```python
from build123d import *

# Parameters (mm, degrees)
F0_W     = 101.6
F0_H     = 25.4
F1_DEPTH = 25.4
F2_DEPTH = 12.7
F3_DEPTH = 63.5
F4_R     = 5.08
F5_SIZE  = 5.08


with BuildPart() as f1:
    # F0 (on Front) → F1 (new body, symmetric)
    with BuildSketch(Plane.XZ):
        Rectangle(F0_W, F0_H)
    extrude(amount=F1_DEPTH, both=True)

    # F0 (on Front) → F2 (join, symmetric)
    with BuildSketch(Plane.XZ):
        Polygon((-50.8, 12.7), (50.8, 12.7), (50.8, 38.1), (0, 38.1), align=None)
    extrude(amount=F2_DEPTH, both=True)

    # F0 (on Front) → F3 (join, symmetric)
    with BuildSketch(Plane.XZ):
        Polygon((50.8, 12.7), (50.8, -12.7), (50.8, -39.22494), (63.5, -39.22494), (63.5, 87.77506), (50.8, 87.77506), (50.8, 38.1), align=None)
    extrude(amount=F3_DEPTH, both=True)

    # F4
    f4_edges = [f1.edges().sort_by_distance(p)[0] for p in [
        (0, 0, 38.1),
    ]]
    fillet(f4_edges, radius=F4_R)

    # F5
    f5_edges = [f1.edges().sort_by_distance(p)[0] for p in [
        (57.15, 63.5, 87.77506),
        (57.15, -63.5, 87.77506),
        (57.15, 63.5, -39.22494),
        (57.15, -63.5, -39.22494),
        (-50.8, 25.4, 0),
        (-50.8, -25.4, 0),
    ]]
    chamfer(f5_edges, length=F5_SIZE)


solid = f1.part
```
Input: part model. Units: mm. Frame: model coordinates. A direction names the side the tool comes from. Coordinates: 2 decimals unless noted, no trailing zeros. Write each loop counter-clockwise with the first axis right and the second up, starting at its lowest first coordinate (ties: lowest second). Pieces come first, ordered by that corner, then holes. Notation, with made-up numbers: (18.5, 51) -> (77.5, 51) arc R27 ccw to (77.5, 78) -> close; hole circle Ø11 at (50, 62.5). An arc over 180 degrees is marked (long way). Write each question's results on one line, items separated by ' | '.
Item 1: Section query B-B on z = 30. Return loops of the section in (x, y).
Conclusion:
outline: (-16.2, -12.7) -> (50.8, -12.7) -> (50.8, -63.5) -> (63.5, -63.5) -> (63.5, 63.5) -> (50.8, 63.5) -> (50.8, 12.7) -> (-16.2, 12.7) -> close
Item 2: Pin query (flat end, axial travel): pin 1 Ø15 at (x, y) = (8.5, -3) entering from -Z; pin 2 Ø6 at (y, z) = (-1, 57) entering from -X; pin 3 Ø8 at (y, z) = (26, -5) entering from -X. Return the tip coordinate at first contact, or that it passes through.
Conclusion:
pin 1: stops at z = -12.7 | pin 2: stops at x = 50.8 | pin 3: stops at x = -49.12
Item 3: Mould query, pull axis Z, two halves, no side actions, for faces 5 (the flat face through (57, -1, -39.225)), 6 (the flat face through (57, 63.5, 25)), 7 (the flat face through (26, 0, 38.1)). Classes: +Z half, -Z half, draft (parallel to the pull), parting line (faces both ways), or undercut.
Conclusion:
face 5: -Z half | face 6: draft | face 7: +Z half
Item 4: Material intervals for probe 1 along X at (y, z) = (10, 57); probe 2 along Y at (x, z) = (47.5, 38), sorted ascending.
Conclusion:
probe 1: x = 50.8 to 63.5 | probe 2: y = -12.7 to 12.7
Item 5: Section query C-C on y = 5.5. Return loops of the section in (x, z), plus the area to 3 significant figures.
Conclusion:
outline: (-50.8, -12.7) -> (50.8, -12.7) -> (50.8, -39.22) -> (63.5, -39.22) -> (63.5, 87.78) -> (50.8, 87.78) -> (50.8, 38.1) -> (1.2, 38.1) arc R5.08 ccw to (-1.07, 37.56) -> (-50.8, 12.7) -> close | area: 6,130 mm^2
Item 6: Set-up query: faces 1 (the flat face through (2, 25.4, 0)), 2 (the flat face through (-1, -19, 12.7)), 3 (the flat face through (2, -25.4, 0)), 4 (the flat face through (-1, 0, -12.7)). Return all of +Z, -Z, +X, -X, +Y, -Y with unobstructed straight access to the full face (end or side cutting, diameter ignored); none if empty.
Conclusion:
face 1: +Z, -Z, -X, +Y | face 2: +Z, -X, -Y | face 3: +Z, -Z, -X, -Y | face 4: -Z, -X, +Y, -Y
Item 7: Section query A-A on x = -41.5. Return loops of the section in (y, z), plus the area to 3 significant figures.
Conclusion:
outline: (-25.4, -12.7) -> (25.4, -12.7) -> (25.4, 12.7) -> (12.7, 12.7) -> (12.7, 17.35) -> (-12.7, 17.35) -> (-12.7, 12.7) -> (-25.4, 12.7) -> close | area: 1,410 mm^2
Item 8: Section query D-D on z = 1.5. Return loops of the section in (x, y).
Conclusion:
outline: (-50.8, -20.32) -> (-45.72, -25.4) -> (50.8, -25.4) -> (50.8, -63.5) -> (63.5, -63.5) -> (63.5, 63.5) -> (50.8, 63.5) -> (50.8, 25.4) -> (-45.72, 25.4) -> (-50.8, 20.32) -> close
